```python
from build123d import *

# Parameters (mm, degrees)
SKETCH1_W           = 10.2
SKETCH1_H           = 16.8
SKETCH1_W_2         = 6.2
SKETCH1_H_2         = 14.1
BOSS_EXTRUDE1_DEPTH = 3
SKETCH2_W           = 6.2
SKETCH2_H           = 2
CUT_EXTRUDE1_DEPTH  = 25.4
SKETCH3_W           = 10.2
SKETCH3_H           = 16.8
BOSS_EXTRUDE2_DEPTH = 2
SKETCH4_R           = 14
SKETCH4_R_2         = 12
BOSS_EXTRUDE4_DEPTH = 5
SKETCH5_R           = 14
BOSS_EXTRUDE5_DEPTH = 2
SKETCH6_W           = 6.2
SKETCH6_H           = 3
CUT_EXTRUDE2_DEPTH  = 7.62


with BuildPart() as part:
    # Sketch1 → Boss-Extrude1 (new body)
    with BuildSketch(Plane(origin=(0, 0, 0), x_dir=(1, 0, 0), z_dir=(0, 1, 0))):
        with Locations((-29.627149571, -6.071905286)):
            Rectangle(SKETCH1_W, SKETCH1_H)
        with Locations((-29.627149571, -5.421905286)):
            Rectangle(SKETCH1_W_2, SKETCH1_H_2, mode=Mode.SUBTRACT)
    extrude(amount=BOSS_EXTRUDE1_DEPTH)

    # Sketch2 → Cut-Extrude1 (cut)
    with BuildSketch(Plane.XY.offset(14.471905286)):
        with Locations((-29.627149571, 2)):
            Rectangle(SKETCH2_W, SKETCH2_H)
    extrude(amount=-CUT_EXTRUDE1_DEPTH, mode=Mode.SUBTRACT)

    # Sketch3 → Boss-Extrude2 (add)
    with BuildSketch(Plane.XZ):
        with Locations((-29.627149571, 6.071905286)):
            Rectangle(SKETCH3_W, SKETCH3_H)
    extrude(amount=BOSS_EXTRUDE2_DEPTH)

    # Sketch4 → Boss-Extrude4 (add)
    with BuildSketch(Plane.XZ.offset(2)):
        with Locations(Location((-29.627149571, 3.222245286, 0), (0, 0, 270))):
            Circle(SKETCH4_R)
        with Locations((-29.627149571, 3.222245286)):
            Circle(SKETCH4_R_2, mode=Mode.SUBTRACT)
    extrude(amount=-BOSS_EXTRUDE4_DEPTH)

    # Sketch5 → Boss-Extrude5 (add)
    with BuildSketch(Plane.XZ.offset(2)):
        with Locations(Location((-29.627149571, 3.222245286, 0), (0, 0, 270))):
            Circle(SKETCH5_R)
    extrude(amount=-BOSS_EXTRUDE5_DEPTH)

    # Sketch6 → Cut-Extrude2 (cut)
    with BuildSketch(Plane.XY.offset(14.471905286)):
        with Locations((-29.627149571, 1.5)):
            Rectangle(SKETCH6_W, SKETCH6_H)
    extrude(amount=CUT_EXTRUDE2_DEPTH, mode=Mode.SUBTRACT)

    # Fillet2: read off the stored shape, not the designer's step
    # Fillet2 outline → Fillet2 (revolve, cut)
    with BuildSketch(Plane(origin=(-29.627149571, 0, 3.222245286), x_dir=(1, 0, 0), z_dir=(0, 0, 1))):
        with BuildLine():
            Line((14, -2), (14, 0))
            ThreePointArc((14, 0), (13.414213562, -1.414213562), (12, -2))
            Line((12, -2), (14, -2))
        make_face()
    revolve(axis=Axis((-29.627149571, 0, 3.222245286), (0, 1, 0)), mode=Mode.SUBTRACT)


solid = part.part
```
Here's how the part is built. I have some questions about the finished solid (model axes, mm). A direction names the side the tool comes from. Give positions to 0.01 mm unless a question says otherwise; leave off trailing zeros. Loops run counter-clockwise (first coordinate to the right, second up) from the corner with the lowest first, then second, coordinate; pieces in that order, holes last. Notation, with made-up numbers: M -26,-18 L 3,-18 A5 cw 3,-14 Z; hole C -3.5,70.25 d4. An arc over 180 degrees is marked long. Use one line per item in the form item = value. Start each with the question number.
Q1. I need wall thicknesses on line 1 along X through (y, z) = (1.15, 11.75); line 2 along X through (y, z) = (0.05, 10.5); line 3 along Z through (x, y) = (-30.75, 0.55). Which ranges of each line are inside material? Lowest first, please.
Q2. If we section it at A-A (y = 0.6): Write out the boundary of the cut face in (x, z), then the cut area to 3 significant figures.
Q3. If we section it at B-B (y = 2.55): Write out the boundary of the cut face in (x, z).
Q4. Which directions (+Z, -Z, +X, -X, +Y, -Y) give clear straight access to the entire face, cutting with the end or side of a thin tool? Please do faces 5 (the flat face through (-32.727, 1, 16)), 6 (the flat face through (-30, 0, 6)), 7 (the flat face through (-29, -2, 3)).
Q5. Thinking about a two-plate mould opening in Z: for faces 1 (the flat face through (-30, 1, 13)), 2 (the cylindrical face through (-30.199, 1.479, -10.766)), 3 (the flat face through (-34.727, 2, 6)), 4 (the flat face through (-29.7, 0.5, 12.472)), which applies, +Z half, -Z half, draft (parallel to the pull), parting line (faces both ways), or undercut?
Q6. Will these pins go through, and if not, where does the flat tip stop? pin 1 Ø3 at (y, z) = (1.5, 13.5) entering from +X; pin 2 Ø1.5 at (x, y) = (-25.5, -0.5) entering from -Z; pin 3 Ø1.5 at (y, z) = (1, 8) entering from -X; pin 4 Ø11.5 at (x, z) = (-25, -2.5) entering from +Y.
Taken from the geometry:
q1.line_1 = -40.73 to -38.07, -34.73 to -32.73, -26.53 to -24.53, -21.18 to -18.52
q1.line_2 = -41.59 to -39.17, -34.73 to -32.73, -26.53 to -24.53, -20.09 to -17.67
q1.line_3 = -10.73 to -8.73, -2.33 to -1.63, 12.47 to 14.47
q2.outline = M -33.8,14.47 A12 cw -32.73,14.81 L -32.73,16.87 A14 ccw long -26.53,16.87 L -26.53,14.81 A12 cw -25.45,14.47 Z; hole M -34.73,-2.33 L -34.73,14.08 A12 ccw long -24.53,14.08 L -24.53,-2.33 Z; hole M -32.73,-1.63 L -26.53,-1.63 L -26.53,12.47 L -32.73,12.47 Z
q2.area = 234 mm^2
q3.outline = M -34.73,-2.33 L -32.73,-2.33 L -32.73,14.47 L -33.8,14.47 A12 cw -32.73,14.81 L -32.73,16.87 A14 ccw long -26.53,16.87 L -26.53,14.81 A12 cw -25.45,14.47 L -26.53,14.47 L -26.53,-2.33 L -24.53,-2.33 L -24.53,14.08 A12 cw long -34.73,14.08 Z
q4.face_5 = +Z, +Y
q4.face_6 = +Y
q4.face_7 = +Z, -Z, +X, -X, -Y
q5.face_1 = draft
q5.face_2 = parting line
q5.face_3 = undercut
q5.face_4 = undercut
q6.pin_1 = -18.72
q6.pin_2 = -10.34
q6.pin_3 = -43.04
q6.pin_4 = 3
